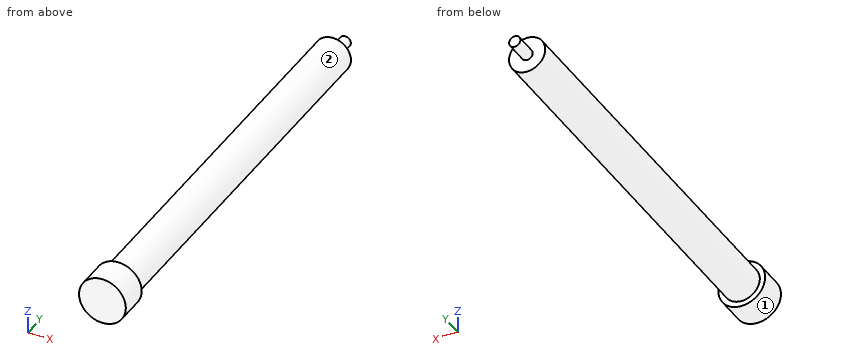
```python
from build123d import *

# Parameters (mm, degrees)
SKETCH1_R           = 7.62
BOSS_EXTRUDE1_DEPTH = 622.3
SKETCH2_R           = 24.511
BOSS_EXTRUDE2_DEPTH = 590.55
SKETCH3_R           = 31.75
BOSS_EXTRUDE3_DEPTH = 40.64


with BuildPart() as part:
    # Sketch1 → Boss-Extrude1 (new body)
    with BuildSketch(Plane(origin=(0, 0, 0), x_dir=(1, 0, 0), z_dir=(0, 1, 0))):
        Circle(SKETCH1_R)
    extrude(amount=BOSS_EXTRUDE1_DEPTH)

    # Sketch2 → Boss-Extrude2 (add)
    with BuildSketch(Plane.XZ):
        Circle(SKETCH2_R)
    extrude(amount=-BOSS_EXTRUDE2_DEPTH)

    # Sketch3 → Boss-Extrude3 (add)
    with BuildSketch(Plane.XZ):
        Circle(SKETCH3_R)
    extrude(amount=-BOSS_EXTRUDE3_DEPTH)


solid = part.part
```
Check sheet for the modelled part. Datum: model origin and axes. Units: mm. Face numbers are marked on the shaded views. A direction names the side the tool comes from. Round coordinates to 2 decimals unless told otherwise and drop trailing zeros. Loops run counter-clockwise (first coordinate to the right, second up) from the corner with the lowest first, then second, coordinate; pieces in that order, holes last. Notation, with made-up numbers: (14, -20) -> (42, -20) arc R9 cw to (42, -8) -> close; hole circle Ø7 at (42, 81). An arc over 180 degrees is marked (long way). Answer in a Markdown table with one row per item.
Q1. Go/stop test with flat-tipped pins: P1, Ø4, axis at x = -5.5, z = 25, coming from the -Y side; P2, Ø12, axis at y = 186.5, z = 8.5, coming from the +X side; P3, Ø8, axis at x = 22, y = 403.5, coming from the +Z side; P4, Ø10, axis at x = 12.5, y = 195.5, coming from the +Z side. Record where each tip stops, or that it passes through.
Data:
| item | result |
|---|---|
| P1 | stops at y = 0 |
| P2 | stops at x = 24.38 |
| P3 | stops at z = 16.64 |
| P4 | stops at z = 23.34 |
Q2. Sectioned sample at C-C on y = 350. Enter the section's corners in (x, z), then the cut area to 3 significant figures.
Data:
| item | result |
|---|---|
| outline | circle Ø49.02 at (0, 0) |
| area | 1,890 mm^2 |
Q3. Thickness scan on L1, parallel to Y at x = 9.5, z = 6.5; L2, parallel to X at y = 188.5, z = 1.5; L3, parallel to Y at x = -27.5, z = 8. Record the ranges inside material, lowest first.
Data:
| item | result |
|---|---|
| L1 | y = 0 to 590.55 |
| L2 | x = -24.47 to 24.47 |
| L3 | y = 0 to 40.64 |
Q4. Sectioned sample at B-B on z = 0. Enter the section's corners in (x, y).
Data:
| item | result |
|---|---|
| outline | (-31.75, 0) -> (31.75, 0) -> (31.75, 40.64) -> (24.51, 40.64) -> (24.51, 590.55) -> (7.62, 590.55) -> (7.62, 622.3) -> (-7.62, 622.3) -> (-7.62, 590.55) -> (-24.51, 590.55) -> (-24.51, 40.64) -> (-31.75, 40.64) -> close |
Q5. Set-up check for the marked faces 1 and 2: record each of +Z, -Z, +X, -X, +Y, -Y from which the full face is reachable in a straight line by a thin tool's end or side.
Data:
| item | result |
|---|---|
| face 1 | +Y, -Y |
| face 2 | +Y |
Q6. Sectioned sample at A-A on x = 0. Enter the section's corners in (y, z), then the cut area to 3 significant figures.
Data:
| item | result |
|---|---|
| outline | (0, -31.75) -> (40.64, -31.75) -> (40.64, -24.51) -> (590.55, -24.51) -> (590.55, -7.62) -> (622.3, -7.62) -> (622.3, 7.62) -> (590.55, 7.62) -> (590.55, 24.51) -> (40.64, 24.51) -> (40.64, 31.75) -> (0, 31.75) -> close |
| area | 30,000 mm^2 |
